Autodesk Inventor part; units mm, degrees
ref_plane "ULC_ULG" through (18, 0, 0) normal (1, 0, 0) x (0, 0, -1)
ref_plane "YZ Plane" through (0, 0, 0) normal (1, 0, 0) x (0, 1, 0)
ref_plane "XZ Plane" through (0, 0, 0) normal (0, 1, 0) x (-1, 0, 0)
sketch "Sketch1" plane through (0, 0, 0) normal (1, 0, 0) x (0, 1, 0)
  line L0 (0, -9) -> (0, 26)
  line L1 (0, 21) -> (-11, 21)
  line L2 (-11, 21) -> (-11, -4)
  line L3 (-11, -4) -> (-4, -4)
  line L4 (-4, -4) -> (-4, -2)
  line L5 (-4, -2) -> (-6.25, -2)
  line L6 (-6.25, -2) -> (-6.25, 0)
  line L7 (-6.25, 0) -> (0, 0)
  line L8 (0, 21) -> (11, 21)
  line L9 (11, 21) -> (11, -4)
  line L10 (11, -4) -> (4, -4)
  line L11 (4, -4) -> (4, -2)
  line L12 (4, -2) -> (6.25, -2)
  line L13 (6.25, -2) -> (6.25, 0)
  line L14 (6.25, 0) -> (0, 0)
  dimension "d1" = 22
  dimension "d2" = 25
  dimension "d3" = 12.5
  dimension "d4" = 8
  dimension "d5" = 4
  dimension "d6" = 2
extrude "Extrusion1" add sketch "Sketch1" along normal blind 18
fillet "Fillet1" radius 5 4 edges at (0, -11, 8.5) (18, -11, 8.5) (18, 11, 8.5) (0, 11, 8.5)
sketch "Sketch2" plane through (0, 0, 0) normal (0, 1, 0) x (-1, 0, 0)
  line L0 (-18, 0) -> (-18, 21) construction
  line L1 (-5, 21) -> (-13, 21) construction
  line L2 (-9, 21) -> (-9, -4)
  line L3 (0, -4) -> (-18, -4) construction
  line L4 (0, 0) -> (0, 0) construction
  arc A0 (0, 6.3589) -> (-18, 6.3589) centre (-9, 2) ccw
  arc A1 (0, 14) -> (-18, 14) centre (-9, 2) ccw
  line L5 (-18, 14) -> (-18, 6.3589)
  line L6 (0, 6.3589) -> (0, 14)
  line L7 (0, 14) -> (0, 6.3589)
  line L8 (-18, 14) -> (-18, 21)
  line L9 (-18, 21) -> (0, 21)
  line L10 (0, 21) -> (0, 14)
  dimension "d10" = 10
  dimension "d11" = 6
  dimension "d18" = 5
extrude "Extrusion2" cut sketch "Sketch2" against normal mid plane 10 contours A1 L6 A0 L2 | L2 A0 L5 A1
extrude "Extrusion3" cut sketch "Sketch2" against normal mid plane 5 contours L9 L10 A1 L2 | L2 A1 L8 L9
ref_plane "ULC_ULG" through (18, 0, 0) normal (1, 0, 0) x (0, 0, -1)
equation "\"d1\" = W_"
equation "\"d2\" = H_"
equation "\"d3\" = ULC_ULG_W1"
equation "\"d4\" = ULC_ULG_W2"
equation "\"d5\" = ULC_ULG_H1"
equation "\"d6\" = ULC_ULG_H2"
equation "\"d7\" = L"
equation "\"d9\" = ULC_a1"
equation "\"d10\" = R"
equation "\"d11\" = RC"
equation "\"d18\" = ULC_ULB_H"
equation "\"d19\" = ULC_ULB_Wmin"
equation "\"d23\" = ULC_ULB_W1"
equation "\"ULC_ULB_H\" = 5"
equation "\"W_\" = 22"
equation "\"L\" = 18"
equation "\"H_\" = 25"
equation "\"RC\" = 6"
equation "\"R\" = 10"
equation "\"ULC_ULB_Wmin\" = 10"
equation "\"ULC_ULB_W1\" = 5"
equation "\"ULC_ULG_W1\" = 12.5"
equation "\"ULC_ULG_W2\" = 8"
equation "\"ULC_ULG_H1\" = 4"
equation "\"ULC_ULG_H2\" = 2"
equation "\"ULC_a1\" = 5"
properties part number "\"ULC 1001\"" material "DIN 1.2344"
CAD build for the part. Positions are in the model's coordinates, mm. A direction names the side the tool comes from. Round coordinates to 2 decimals unless told otherwise and drop trailing zeros. Loops run counter-clockwise (first coordinate to the right, second up) from the corner with the lowest first, then second, coordinate; pieces in that order, holes last. Notation, with made-up numbers: M 37,-35.5 L 70,-35.5 A13 cw 70,-18.5 Z; hole C 24.5,78.5 d9. An arc over 180 degrees is marked long. Use a Markdown table: item, result. Add a question column.
(1) Cut at C-C (z = 0.5). Give the cut face in (x, y).
(2) Which spindle directions (+Z, -Z, +X, -X, +Y, -Y) get a long thin tool onto all of the face, cutting with end or side? Do faces 1 (the face through (9, -5, -2)), 2 (the face through (9, -4, -3)), 3 (the face through (9, 4, 17)), 4 (the face through (9, -2.5, 18)). Say none if no direction does.
(3) Cut at A-A (z = 13.5). Give the cut face in (x, y), and give its area (3 significant figures).
(4) Drill centre lines: line 1 (Z direction, x = 7, y = 6); line 2 (Y direction, x = 6.75, z = -2.25); line 3 (Z direction, x = 5.25, y = 3). Where is each one in solid material? Low to high.
(5) Pull direction Y, two halves, no side cores. Call faces 5 (the face through (9, -4, 17)), 6 (the face through (9, 8, -4)), 7 (the face through (1, -9, 9)): +Y half, -Y half, draft (parallel to the pull), parting line (faces both ways), or undercut.
(6) Cut at B-B (x = 4.25). Give the cut face in (y, z), and give its area (3 significant figures).
(7) Cut at D-D (z = 18.25). Give the cut face in (x, y), and give its area (3 significant figures).
Geometry says:
| question | item | result |
|---|---|---|
| 1 | outline | M 0,-6 A5 ccw 5,-11 L 13,-11 A5 ccw 18,-6 L 18,6 A5 ccw 13,11 L 5,11 A5 ccw 0,6 Z |
| 2 | face 1 | +X, -X |
| 2 | face 2 | -Z, +X, -X |
| 2 | face 3 | none |
| 2 | face 4 | +Z, +X, -X |
| 3 | outline | M 0,-6 A5 ccw 5,-11 L 13,-11 A5 ccw 18,-6 L 18,-5 L 0,-5 Z; M 0,5 L 18,5 L 18,6 A5 ccw 13,11 L 5,11 A5 ccw 0,6 Z |
| 3 | area | 195 mm² |
| 4 | line 1 | z = -4 to -2, 0 to 21 |
| 4 | line 2 | y = -11 to -4, 4 to 11 |
| 4 | line 3 | z = 0 to 11.27, 16.52 to 21 |
| 5 | face 5 | undercut |
| 5 | face 6 | draft |
| 5 | face 7 | -Y half |
| 6 | outline | M -10.94,-4 L -4,-4 L -4,-2 L -6.25,-2 L -6.25,0 L 6.25,0 L 6.25,-2 L 4,-2 L 4,-4 L 10.94,-4 L 10.94,21 L 2.5,21 L 2.5,16.23 L 5,16.23 L 5,10.8 L -5,10.8 L -5,16.23 L -2.5,16.23 L -2.5,21 L -10.94,21 Z |
| 6 | area | 428 mm² |
| 7 | outline | M 0,-6 A5 ccw 5,-11 L 13,-11 A5 ccw 18,-6 L 18,-2.5 L 0,-2.5 Z; M 0,2.5 L 18,2.5 L 18,6 A5 ccw 13,11 L 5,11 A5 ccw 0,6 Z |
| 7 | area | 285 mm² |
